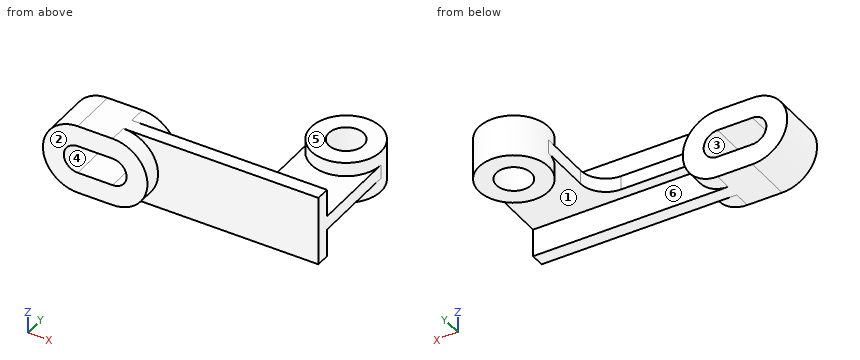
from build123d import *

# Parameters (mm, degrees)
BOSS_EXTRUDE10_DEPTH       = 22.5
BOSS_EXTRUDE10_DEPTH_BACK  = 12.5
BOSS_EXTRUDE11_DEPTH       = 10
BOSS_EXTRUDE12_DEPTH       = 18
BOSS_EXTRUDE13_DEPTH       = 5
BOSS_EXTRUDE13_DEPTH_BACK  = 5
BOSS_EXTRUDE14_START       = -15
BOSS_EXTRUDE14_OUTLINE_R   = 25
BOSS_EXTRUDE14_OUTLINE_R_2 = 12.5
BOSS_EXTRUDE14_DEPTH       = 30


# Read off the part's stored shape, not the designer's step: Boss-Extrude14
with BuildPart() as part:
    # Sketch1 → Boss-Extrude10 (new, two sides: drawn at the far end of the back side and taken through both)
    with BuildSketch(Plane(origin=(0, 0, 0), x_dir=(1, 0, 0), z_dir=(0, 1, 0)).offset(-BOSS_EXTRUDE10_DEPTH_BACK)):
        with BuildLine():
            Line((-70.624644485, -25), (-45.624644485, -25))
            ThreePointArc((-45.624644485, -25), (-20.624644485, 0), (-45.624644485, 25))
            Line((-45.624644485, 25), (-70.624644485, 25))
            ThreePointArc((-70.624644485, 25), (-95.624644485, 0), (-70.624644485, -25))
        make_face()
        with BuildLine():
            ThreePointArc((-45.624644485, -10), (-35.624644485, 0), (-45.624644485, 10))
            Line((-45.624644485, 10), (-70.624644485, 10))
            ThreePointArc((-70.624644485, 10), (-80.624644485, 0), (-70.624644485, -10))
            Line((-70.624644485, -10), (-45.624644485, -10))
        make_face(mode=Mode.SUBTRACT)
    extrude(amount=BOSS_EXTRUDE10_DEPTH + BOSS_EXTRUDE10_DEPTH_BACK)

    # Sketch1<6> → Boss-Extrude11 (add)
    with BuildSketch(Plane(origin=(0, 0, 0), x_dir=(1, 0, 0), z_dir=(0, 1, 0))):
        with BuildLine():
            ThreePointArc((-21.129747057, -5), (-29.813256184, -19.364916731), (-45.624644485, -25))
            Line((-45.624644485, -25), (94.375355515, -25))
            Line((94.375355515, -25), (94.375355515, -5))
            Line((94.375355515, -5), (-21.129747057, -5))
        make_face()
        with BuildLine():
            Line((94.375355515, 25), (-45.624644485, 25))
            ThreePointArc((-45.624644485, 25), (-29.813256184, 19.364916731), (-21.129747057, 5))
            Line((-21.129747057, 5), (94.375355515, 5))
            Line((94.375355515, 5), (94.375355515, 25))
        make_face()
    extrude(amount=BOSS_EXTRUDE11_DEPTH)

    # Sketch1<7> → Boss-Extrude12 (add)
    with BuildSketch(Plane(origin=(0, 0, 0), x_dir=(1, 0, 0), z_dir=(0, 1, 0))):
        with BuildLine():
            Line((94.375355515, 5), (-21.129747057, 5))
            ThreePointArc((-21.129747057, 5), (-20.624644485, 0), (-21.129747057, -5))
            Line((-21.129747057, -5), (94.375355515, -5))
            Line((94.375355515, -5), (94.375355515, 5))
        make_face()
    extrude(amount=BOSS_EXTRUDE12_DEPTH)

    # Sketch2 → Boss-Extrude13 (add, two sides: drawn at the far end of the back side and taken through both)
    with BuildSketch(Plane.XY.offset(-BOSS_EXTRUDE13_DEPTH_BACK)):
        with BuildLine():
            ThreePointArc((44.375355515, 36), (39.103277576, 23.272077939), (26.375355515, 18))
            Line((26.375355515, 18), (94.375355515, 18))
            Line((94.375355515, 18), (94.375355515, 73.5))
            ThreePointArc((94.375355515, 73.5), (69.375355515, 48.5), (44.375355515, 73.5))
            Line((44.375355515, 73.5), (44.375355515, 36))
        make_face()
    extrude(amount=BOSS_EXTRUDE13_DEPTH + BOSS_EXTRUDE13_DEPTH_BACK)

    # Boss-Extrude14 outline → Boss-Extrude14 (add)
    with BuildSketch(Plane.XY.offset(BOSS_EXTRUDE14_START)):
        with Locations((69.375355515, 73.5)):
            Circle(BOSS_EXTRUDE14_OUTLINE_R)
        with Locations((69.375355515, 73.5)):
            Circle(BOSS_EXTRUDE14_OUTLINE_R_2, mode=Mode.SUBTRACT)
    extrude(amount=BOSS_EXTRUDE14_DEPTH)


solid = part.part
Model file for the job. Use its own axes, mm. Face numbers are marked on the shaded views. A direction names the side the tool comes from. Round coordinates to 2 decimals unless told otherwise and drop trailing zeros. Order: outer loops, then holes, each group sorted by start corner. A loop starts at its lowest first (then second) coordinate and runs counter-clockwise, first axis right, second up.
(1) Band-saw the part on A-A (x = -58.5). List the corners of the cut face in (y, z), then the cut area to 3 significant figures.
(2) Band-saw the part on D-D (z = -19). List the corners of the cut face in (x, y).
(3) Band-saw the part on C-C (y = 15). List the corners of the cut face in (x, z).
(4) 3-axis set-ups, long thin cutter, end or side, ignore diameter. For the marked faces 4, 5 and 6: which of +Z, -Z, +X, -X, +Y, -Y reach the whole face in a straight line?
(5) Pin check, flat tips, straight feed: pin 1 (8 mm diameter, centred on y = 52, z = 0, fed in from -X); pin 2 (8 mm diameter, centred on x = 10, z = -0.5, fed in from +Y); pin 3 (3 mm diameter, centred on x = 31, z = 16.5, fed in from -Y). Stop position of each tip, or through.
(6) Pull direction Y, two halves, no side cores. Call the marked faces 1, 2 and 3: released by +Y, released by -Y, zero draft, split by the parting line, or undercut.
(7) Drill centre lines: line 1 (Z direction, x = -62, y = 8); line 2 (X direction, y = 73, z = 0); line 3 (Z direction, x = 74, y = 49.5). Where is each one in solid material? Low to high.
(8) Band-saw the part on B-B (z = 0). List the corners of the cut face in (x, y), then the cut area to 3 significant figures.
Verdict:
1. outline: (-12.5, -25) - (22.5, -25) - (22.5, -10) - (-12.5, -10) - close; (-12.5, 10) - (22.5, 10) - (22.5, 25) - (-12.5, 25) - close
1. area: 1,050 mm2
2. outline: (-86.87, -12.5) - (-29.38, -12.5) - (-29.38, 0) - (94.38, 0) - (94.38, 10) - (-29.38, 10) - (-29.38, 22.5) - (-86.87, 22.5) - close
3. outline: (-70.62, -25) - (-45.62, -25) arc R25 ccw to (-21.13, -5) - (94.38, -5) - (94.38, 5) - (-21.13, 5) arc R25 ccw to (-45.62, 25) - (-70.62, 25) arc R25 ccw to start; hole (-70.62, -10) - (-45.62, -10) arc R10 ccw to (-45.62, 10) - (-70.62, 10) arc R10 ccw to start
4. face 4: +Y, -Y
4. face 5: +Z, +X, -X, +Y
4. face 6: -Z, +X
5. pin 1: stops at x = 44.38
5. pin 2: stops at y = 18
5. pin 3: stops at y = 0
6. face 1: undercut
6. face 2: released by -Y
6. face 3: zero draft
7. line 1: z = -25 to -10, 10 to 25
7. line 2: x = 44.38 to 56.89, 81.87 to 94.38
7. line 3: z = -15 to 15
8. outline: (-95.62, -12.5) - (-80.62, -12.5) - (-80.62, 22.5) - (-95.62, 22.5) - close; (-35.62, -12.5) - (-20.62, -12.5) - (-20.62, 0) - (94.38, 0) - (94.38, 73.5) arc R25 ccw to (44.38, 73.5) - (44.38, 36) arc R18 cw to (26.38, 18) - (-20.62, 18) - (-20.62, 22.5) - (-35.62, 22.5) - close; hole circle Ø25 at (69.38, 73.5)
8. area: 6,460 mm2
